```python
from build123d import *

# Parameters (mm, degrees)
SKETCH1_R           = 3.5
BOSS_EXTRUDE1_DEPTH = 4
SKETCH2_R           = 2
BOSS_EXTRUDE2_DEPTH = 8
CUT_EXTRUDE1_DEPTH  = 2.5
FILLET1_R           = 0.5
CHAMFER1_SIZE       = 0.2


with BuildPart() as part:
    # Sketch1 → Boss-Extrude1 (new body)
    with BuildSketch(Plane.XY):
        Circle(SKETCH1_R)
    extrude(amount=BOSS_EXTRUDE1_DEPTH)

    # Sketch2 → Boss-Extrude2 (add)
    with BuildSketch(Plane.XY.offset(4)):
        Circle(SKETCH2_R)
    extrude(amount=BOSS_EXTRUDE2_DEPTH)

    # Sketch3 → Cut-Extrude1 (cut)
    with BuildSketch(Plane(origin=(0, 0, 0), x_dir=(-1, 0, 0), z_dir=(0, 0, -1))):
        Polygon((2.020725942, 0), (1.010362971, 1.75), (-1.010362971, 1.75), (-2.020725942, 0), (-1.010362971, -1.75), (1.010362971, -1.75), align=None)
    extrude(amount=-CUT_EXTRUDE1_DEPTH, mode=Mode.SUBTRACT)

    # Fillet1
    fillet1_edges = [part.edges().sort_by_distance(p)[0] for p in [
        (-1.515544457, -0.875, 0),
        (-1.515544457, 0.875, 0),
        (0, 1.75, 0),
        (1.515544457, 0.875, 0),
        (1.515544457, -0.875, 0),
        (0, -1.75, 0),
        (-3.5, 0, 0),
        (-3.5, 0, 4),
        (-2, 0, 4),
    ]]
    fillet(fillet1_edges, radius=FILLET1_R)

    # Chamfer1
    chamfer1_edges = [part.edges().sort_by_distance(p)[0] for p in [
        (-2, 0, 12),
    ]]
    chamfer(chamfer1_edges, length=CHAMFER1_SIZE)


solid = part.part
```
Check sheet for the modelled part. Datum: model origin and axes. Units: mm. A direction names the side the tool comes from. Round coordinates to 2 decimals unless told otherwise and drop trailing zeros. Write each loop counter-clockwise with the first axis right and the second up, starting at its lowest first coordinate (ties: lowest second). Pieces come first, ordered by that corner, then holes. Notation, with made-up numbers: M -4.75,-32 L 12.25,-32 A29 ccw 12.25,-9 Z; hole C 83,2.5 d9. An arc over 180 degrees is marked long. Write item = value, one per line. Start each with the question number.
1. Section check B-B, the plane z = 2.25. Record the cut outline in (x, y), then the cut area to 3 significant figures.
2. Section check A-A, the plane x = 0. Record the cut outline in (y, z), then the cut area to 3 significant figures.
3. Tool access check on faces 4 (the flat face through (0, 1.75, 1)), 5 (the flat face through (2, -2, 0)). Record the directions out of +Z, -Z, +X, -X, +Y, -Y that give a thin tool (end or side, any length) a straight path to the whole face; none if there is none.
4. Release check for a two-part mould opening along X. For faces 1 (the cylindrical face through (-1.64, 0.97, 0.14)), 2 (the cylindrical face through (0, -2, 8)), 3 (the flat face through (-2, 2, 4)) record: pulls with the +X half, pulls with the -X half, needs draft (parallel to the pull), parting line crosses it, or undercut.
5. Scan lines: line 1 (Z direction, x = 0.5, y = -2.5); line 2 (Y direction, x = 0.5, z = 1.25); line 3 (Z direction, x = 0, y = -0.5). Record each from-to range of solid material in increasing order. Write a range as [from, to].
6. Section check C-C, the plane z = 6.25. Record the cut outline in (x, y), then the cut area to 3 significant figures.
7. Gauge pin test, flat ends, axial feed: pin 1 (3 mm diameter, centred on y = -0.5, z = 10.5, fed in from +X); pin 2 (2 mm diameter, centred on y = 2, z = 10.5, fed in from +X); pin 3 (1 mm diameter, centred on x = 2, z = 7.5, fed in from -Y). Record the tip position at first contact, or that the pin passes through.
Results found:
q1.outline = C 0,0 d7; hole M -2.02,0 L -1.01,-1.75 L 1.01,-1.75 L 2.02,0 L 1.01,1.75 L -1.01,1.75 Z
q1.area = 27.9 mm^2
q2.outline = M -3.5,0.5 A0.5 ccw -3,0 L -2.25,0 A0.5 ccw -1.75,0.5 L -1.75,2.5 L 1.75,2.5 L 1.75,0.5 A0.5 ccw 2.25,0 L 3,0 A0.5 ccw 3.5,0.5 L 3.5,3.5 A0.5 ccw 3,4 L 2.5,4 A0.5 cw 2,4.5 L 2,11.8 L 1.8,12 L -1.8,12 L -2,11.8 L -2,4.5 A0.5 cw -2.5,4 L -3,4 A0.5 ccw -3.5,3.5 Z
q2.area = 51.0 mm^2
q3.face_4 = -Z
q3.face_5 = -Z, +X, -X, +Y, -Y
q4.face_1 = undercut
q4.face_2 = parting line crosses it
q4.face_3 = needs draft
q5.line_1 = [0, 4]
q5.line_2 = [-3.46, -1.75], [1.75, 3.46]
q5.line_3 = [2.5, 12]
q6.outline = C 0,0 d4
q6.area = 12.6 mm^2
q7.pin_1 = 2
q7.pin_2 = 1.73
q7.pin_3 = -1.32
